```python
from build123d import *

# Parameters (mm, degrees)
SKETCH1_R           = 3.9
BOSS_EXTRUDE1_DEPTH = 44
BOSS_EXTRUDE2_START = 5
SKETCH6_R           = 3.9
BOSS_EXTRUDE2_DEPTH = 5
CUT_EXTRUDE1_DEPTH  = 8
CUT_EXTRUDE2_DEPTH  = 15


# Read off the part's stored shape, not the designer's step: 1/4-20 Machine Threads Stud2, 1/4-20 Machine Threads Stud4
with BuildPart() as part:
    # Sketch1 → Boss-Extrude1 (new body)
    with BuildSketch(Plane(origin=(0, 0, 0), x_dir=(1, 0, 0), z_dir=(0, 1, 0))):
        with Locations(Location((0, 0, 0), (0, 0, 270))):
            Circle(SKETCH1_R)
    extrude(amount=BOSS_EXTRUDE1_DEPTH)

    # 1/4-20 Machine Threads Stud2 outline → 1/4-20 Machine Threads Stud2 (revolve, cut)
    with BuildSketch(Plane.XY):
        Polygon((3.9, 44), (2.41935, 44), (3.175, 43.24435), (3.175, 37), (3.9, 37), align=None)
    revolve(axis=Axis((0, 0, 0), (0, 1, 0)), mode=Mode.SUBTRACT)

    # Sketch6 → Boss-Extrude2 (add)
    with BuildSketch(Plane.XZ.offset(BOSS_EXTRUDE2_START)):
        with Locations(Location((0, 0, 0), (0, 0, 270))):
            Circle(SKETCH6_R)
    extrude(amount=-BOSS_EXTRUDE2_DEPTH)

    # 1/4-20 Machine Threads Stud4 outline → 1/4-20 Machine Threads Stud4 (revolve, cut)
    with BuildSketch(Plane.XY):
        Polygon((2.41935, -5), (3.9, -5), (3.9, 5), (3.175, 5), (3.175, -4.24435), align=None)
    revolve(axis=Axis((0, 0, 0), (0, 1, 0)), mode=Mode.SUBTRACT)

    # Sketch10 → Cut-Extrude1 (cut)
    with BuildSketch(Plane.XZ.offset(5)):
        with BuildLine():
            Line((-1.269821024, 0.798470142), (1.269821024, 0.798470142))
            ThreePointArc((1.269821024, 0.798470142), (0, -1.5), (-1.269821024, 0.798470142))
        make_face()
    extrude(amount=-CUT_EXTRUDE1_DEPTH, mode=Mode.SUBTRACT)

    # Sketch11 → Cut-Extrude2 (cut)
    with BuildSketch(Plane.XZ.offset(5)):
        with BuildLine():
            Line((-1.839869815, 0.784142248), (0.828669593, 1.820249078))
            ThreePointArc((0.828669593, 1.820249078), (0.723885911, -1.86440049), (-1.839869815, 0.784142248))
        make_face()
    extrude(amount=-CUT_EXTRUDE2_DEPTH, mode=Mode.SUBTRACT)


solid = part.part
```
Check sheet for the modelled part. Datum: model origin and axes. Units: mm. A direction names the side the tool comes from. Coordinates: 2 decimals unless noted, no trailing zeros. Write each loop counter-clockwise with the first axis right and the second up, starting at its lowest first coordinate (ties: lowest second). Pieces come first, ordered by that corner, then holes. Notation, with made-up numbers: M 35,1.25 L 68,1.25 A26 ccw 68,27.25 Z; hole C 42.5,40.5 d7. An arc over 180 degrees is marked long. Write item = value, one per line. Start each with the question number.
1. Tool access check on faces 1 (the flat face through (-0.524, 2.395, 1.295)), 2 (the cylindrical face through (-1.5, 20.8, 3.6)), 3 (the cylindrical face through (-0.69, 40.08, 3.1)). Record the directions out of +Z, -Z, +X, -X, +Y, -Y that give a thin tool (end or side, any length) a straight path to the whole face; none if there is none.
2. Thickness scan on probe 1 along X at (y, z) = (7.25, 0); probe 2 along X at (y, z) = (-0.75, 0) (3 decimals); probe 3 along Z at (x, y) = (-0.25, -1.5). Record the ranges inside material, lowest first.
3. Sectioned sample at B-B (y = 24.5). Record the cut outline in (x, z).
4. Mould release check, pull along X, two halves, no side actions. Record for faces 4 (the flat face through (-0.7, -5, 1.4)), 5 (the cylindrical face through (-0.69, 0.31, 3.1)), 6 (the flat face through (0, 10, 0)): pulls with the +X half, pulls with the -X half, needs draft (parallel to the pull), parting line crosses it, or undercut.
5. Sectioned sample at A-A (z = 0). Record the cut outline in (x, y) (3 decimals), then the cut area to 3 significant figures.
6. Go/stop test with flat-tipped pins: pin 1 (1.5 mm diameter, centred on y = 38, z = -3, fed in from +X); pin 2 (1 mm diameter, centred on y = 10, z = -1, fed in from +X). Record where each tip stops, or that it passes through.
The answers:
q1.face_1 = -Y
q1.face_2 = +Y, -Y
q1.face_3 = +Y
q2.probe_1 = -3.9 to -2, 2 to 3.9
q2.probe_2 = -3.175 to -2, 2 to 3.175
q2.probe_3 = -3.17 to -1.98, 1.4 to 3.17
q3.outline = C 0,0 d7.8
q4.face_4 = needs draft
q4.face_5 = parting line crosses it
q4.face_6 = undercut
q5.outline = M -3.9,5 L -3.175,5 L -3.175,-4.244 L -2.419,-5 L -2,-5 L -2,10 L 2,10 L 2,-5 L 2.419,-5 L 3.175,-4.244 L 3.175,5 L 3.9,5 L 3.9,37 L 3.175,37 L 3.175,43.244 L 2.419,44 L -2.419,44 L -3.175,43.244 L -3.175,37 L -3.9,37 Z
q5.area = 296 mm²
q6.pin_1 = 2.24
q6.pin_2 = 3.87
